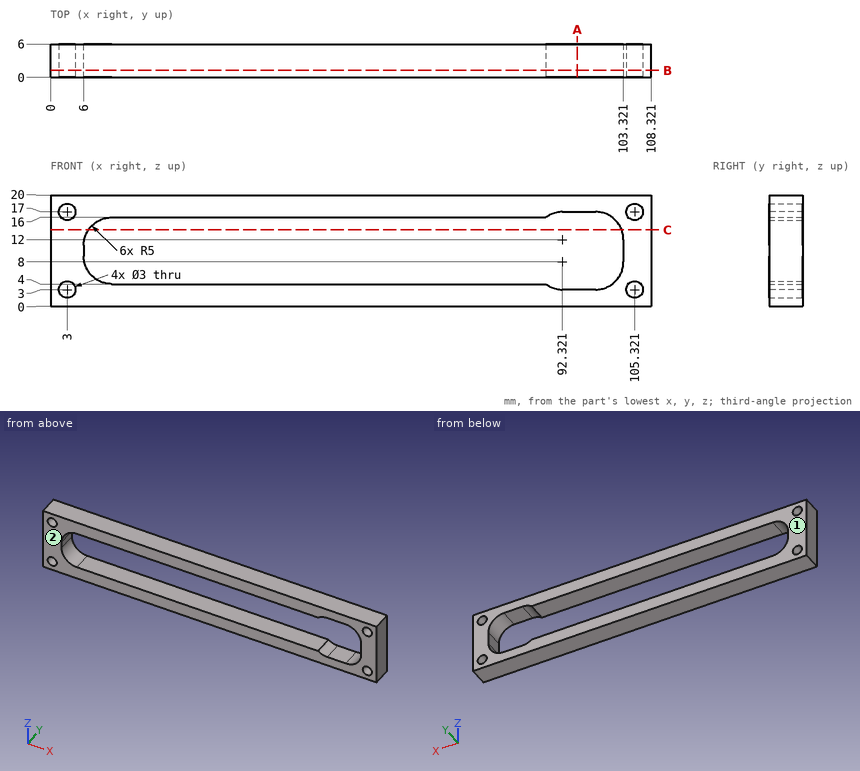
Design review of the part shown in the three views and the two pictorial views. Dimensions are in mm from the part's minimum x, y and z. Round coordinates to 2 decimals unless told otherwise and drop trailing zeros. Write each loop counter-clockwise with the first axis right and the second up, starting at its lowest first coordinate (ties: lowest second). Pieces come first, ordered by that corner, then holes. Notation, with made-up numbers: M -24,77.5 L 23,77.5 A27 ccw 23,108.5 Z; hole C 73.5,2.25 d3. An arc over 180 degrees is marked long. One line per item, written item: value. Start each with the question number.
1. Take a section at C-C on z = 13.75. State the section outline as (x, y) points.
2. Take a section at B-B on y = 1.25. State the section outline as (x, z) points, then the cut area to 3 significant figures.
3. Take a section at A-A on x = 95. State the section outline as (y, z) points.
4. Clearance check with flat-ended pins moving along their axes: P1, Ø5, axis at x = 3, z = 17, coming from the -Y side; P2, Ø1.5, axis at x = 43, z = 5.5, coming from the -Y side. State where each tip first meets the part, or that it passes through.
5. Draft analysis for pull direction Y (two halves, no side actions). For the marked faces 1 and 2, state which applies: pulls with the +Y half, pulls with the -Y half, needs draft (parallel to the pull), parting line crosses it, or undercut.
6. To check wall thickness, follow probe 1 along Z at (x, y) = (18, 4.65); probe 2 along X at (y, z) = (2.9, 15.25) (1 decimal); probe 3 along X at (y, z) = (2.6, 7). State the ranges of each line that lie inside material, in increasing order. Write a range as from..to.
Computed:
1. outline: M 0,0 L 6.82,0 L 6.82,6 L 0,6 Z; M 103,0 L 108.32,0 L 108.32,6 L 103,6 Z
2. outline: M 0,0 L 108.32,0 L 108.32,20 L 0,20 Z; hole C 3,3 d3; hole C 3,17 d3; hole M 6,9 A5 ccw 11,4 L 89.32,4 A5 ccw 92.32,3 L 98.32,3 A5 ccw 103.32,8 L 103.32,12 A5 ccw 98.32,17 L 92.32,17 A5 ccw 89.32,16 L 11,16 A5 ccw 6,11 Z; hole C 105.32,3 d3; hole C 105.32,17 d3
2. area: 966 mm²
3. outline: M 0,0 L 6,0 L 6,3 L 0,3 Z; M 0,17 L 6,17 L 6,20 L 0,20 Z
4. P1: stops at y = 0
4. P2: passes through
5. face 1: pulls with the +Y half
5. face 2: pulls with the -Y half
6. probe 1: z = 0..4, 16..20
6. probe 2: x = 0..8.4, 102.1..108.3
6. probe 3: x = 0..6.42, 103.22..108.32
